from build123d import *

# Parameters (mm, degrees)
CUT_EXTRUDE1_DEPTH = 25.892


with BuildPart() as part:
    # Sketch1 → Revolve1 (revolve)
    with BuildSketch(Plane(origin=(0, 0, 0), x_dir=(0, 0, -1), z_dir=(1, 0, 0))):
        Polygon((0, 0), (0, 18.542), (6.985, 18.542), (6.985, 6.35), (8.89, 6.35), (8.89, 0), (4.7625, 0), (4.7625, -6.35), (0, -6.35), align=None)
    revolve(axis=Axis((0, 0, 0), (0, 1, 0)))

    # Sketch2 → Cut-Extrude1 (cut, through all)
    with BuildSketch(Plane(origin=(0, 18.542, 0), x_dir=(1, 0, 0), z_dir=(0, 1, 0))):
        with BuildLine():
            Line((-7.874, -4.12701151), (-7.874, 4.12701151))
            ThreePointArc((-7.874, 4.12701151), (-8.89, 0), (-7.874, -4.12701151))
        make_face()
        with BuildLine():
            ThreePointArc((8.89, 0), (8.632263898, 2.125116467), (7.874, 4.12701151))
            Line((7.874, 4.12701151), (7.874, -4.12701151))
            ThreePointArc((7.874, -4.12701151), (8.632263898, -2.125116467), (8.89, 0))
        make_face()
    extrude(amount=-CUT_EXTRUDE1_DEPTH, mode=Mode.SUBTRACT)


solid = part.part
Build history of the part. All positions in model axes, mm. A direction names the side the tool comes from. Give positions to 0.01 mm unless a question says otherwise; leave off trailing zeros. Loops run counter-clockwise (first coordinate to the right, second up) from the corner with the lowest first, then second, coordinate; pieces in that order, holes last. Notation, with made-up numbers: (76, 1) - (135, 1) arc R19 ccw to (135, 28) - close; hole circle Ø5 at (38, 8). An arc over 180 degrees is marked (long way). Write item = value, one per line. Start each with the question number.
1) Band-saw the part on D-D on y = 2.25. Give the cut face in (x, z), plus the area to 3 significant figures.
2) Probe probe 1 along Y at (x, z) = (3, 5); probe 2 along Y at (x, z) = (2.75, -7.5); probe 3 along X at (y, z) = (6.75, 0.75). List the from-to ranges inside material, lowest first. Write a range as from..to.
3) Tool access for faces 1 (the cylindrical face through (2.9, -3.22, 3.78)), 2 (the flat face through (6, 6.35, -4)), 3 (the flat face through (-7.874, 3, 0)): list every direction of +Z, -Z, +X, -X, +Y, -Y with a clear straight run to the whole face (end or side of a thin tool).
4) Band-saw the part on C-C on y = 14.75. Give the cut face in (x, z) (3 decimals), plus the area to 3 significant figures.
5) Drop flat-ended pins along their axis: pin 1 Ø6 at (y, z) = (12.5, 1) entering from -X (3 decimals); pin 2 Ø4 at (x, y) = (-3.5, 6) entering from -Z; pin 3 Ø5 at (x, y) = (4, 2) entering from +Z. Give the stop position or say it passes through.
Final values:
q1.outline = (-7.87, -4.13) arc R8.89 ccw to (7.87, -4.13) - (7.87, 4.13) arc R8.89 ccw to (-7.87, 4.13) - close
q1.area = 237 mm²
q2.probe_1 = 0..18.54
q2.probe_2 = 0..6.35
q2.probe_3 = -6.94..6.94
q3.face_1 = -Y
q3.face_2 = +Y
q3.face_3 = +Z, -Z, -X, +Y, -Y
q4.outline = circle Ø13.97 at (0, 0)
q4.area = 153 mm²
q5.pin_1 = -6.985
q5.pin_2 = -8.76
q5.pin_3 = 8.76
